Build history of the part. All positions in model axes, mm. A direction names the side the tool comes from. Coordinates: 2 decimals unless noted, no trailing zeros. Loops run counter-clockwise (first coordinate to the right, second up) from the corner with the lowest first, then second, coordinate; pieces in that order, holes last.
Item 1: Mould opens along Z. For faces 3 (the face through (0, 0, -130.5)), 4 (the face through (-5.5, 2.86, -128.46)), 5 (the face through (0, 0, 0)), 6 (the face through (-3.955, -5.158, -129.507)) say: released by +Z, released by -Z, zero draft, split by the parting line, or undercut.
Item 2: 3-axis set-ups, long thin cutter, end or side, ignore diameter. For faces 1 (the face through (-3.955, -5.158, -66.817)), 2 (the face through (-10.74, -2.38, -2.27)): which of +Z, -Z, +X, -X, +Y, -Y reach the whole face in a straight line?
Item 3: Cut at A-A (x = 0). List the corners of the cut face in (y, z).
Item 4: Drill centre lines: line 1 along Z through (x, y) = (-5.5, -5.25); line 2 along Y through (x, z) = (-2, -96); line 3 along Y through (x, z) = (-3.5, -59.5). Where is each one in solid material? Low to high.
Item 5: Flat gauge pins, fed straight in: pin 1 (4 mm diameter, centred on y = 4, z = -30.5, fed in from +X); pin 2 (10 mm diameter, centred on y = 8, z = -60, fed in from -X); pin 3 (5 mm diameter, centred on x = -2, z = -22, fed in from -Y). Where does each tip first touch, or does it go through?
Item 6: Cut at C-C (z = -109). List the corners of the cut face in (x, y).
Autodesk Inventor part; units mm, degrees
ref_plane "YZ Plane" through (0, 0, 0) normal (1, 0, 0) x (0, 1, 0)
ref_plane "XZ Plane" through (0, 0, 0) normal (0, 1, 0) x (-1, 0, 0)
ref_plane "XY Plane" through (0, 0, 0) normal (0, 0, 1) x (1, 0, 0)
sketch "Náčrt2" plane through (0, 0, 0) normal (1, 0, 0) x (0, 1, 0)
  line L0 (0, 0) -> (0, -130.5)
  line L1 (0, 0) -> (11, 0)
  line L2 (11, 0) -> (11, -4)
  line L3 (11, -4) -> (6.5, -4)
  line L4 (6.5, -4) -> (6.5, -127.9)
  line L5 (6.5, -127.9) -> (6.2, -127.9)
  line L6 (6.2, -127.9) -> (6.2, -129)
  line L7 (6.2, -129) -> (6.5, -129)
  line L8 (6.5, -129) -> (6.5, -130.5)
  line L9 (6.5, -130.5) -> (0, -130.5)
  dimension "d0" = 13
  dimension "d1" = 22
  dimension "d3" = 4
  dimension "d4" = 12.4
  dimension "d5" = 1.1
  dimension "d6" = 1.5
  dimension "d11" = 123.9
  dimension "d12" = 130.5
revolve "Rotace1" add sketch "Náčrt2" angle 360 about axis through (0, 0, 0) along (0, 0, -1)
chamfer "Zkosení1" distance 0.5 angle 45 2 edges at (0, -11, 0) (0, -6.5, -130.5)
properties part number "DD_KVD_003_10_B" material "Nerezová ocel"
Filled sheet:
1. face 3: released by -Z
1. face 4: undercut
1. face 5: released by +Z
1. face 6: zero draft
2. face 1: -Z
2. face 2: +Z, -Z
3. outline: (-11, -4) - (-6.5, -4) - (-6.5, -127.9) - (-6.2, -127.9) - (-6.2, -129) - (-6.5, -129) - (-6.5, -130) - (-6, -130.5) - (6, -130.5) - (6.5, -130) - (6.5, -129) - (6.2, -129) - (6.2, -127.9) - (6.5, -127.9) - (6.5, -4) - (11, -4) - (11, -0.5) - (10.5, 0) - (-10.5, 0) - (-11, -0.5) - close
4. line 1: z = -4 to 0
4. line 2: y = -6.18 to 6.18
4. line 3: y = -5.48 to 5.48
5. pin 1: stops at x = 6.18
5. pin 2: stops at x = -5.77
5. pin 3: stops at y = -6.5
6. outline: circle Ø13 at (0, 0)
